Verification items for the finished model (mm, model axes). Give positions to 0.01 mm unless a question says otherwise; leave off trailing zeros. Loops run counter-clockwise (first coordinate to the right, second up) from the corner with the lowest first, then second, coordinate; pieces in that order, holes last. Notation, with made-up numbers: (63.5, -13.5) - (115.5, -13.5) arc R8 cw to (115.5, -0.5) - close; hole circle Ø10 at (46, 59). An arc over 180 degrees is marked (long way). One line per question, with ' | ' between items. Start each with the question number.
1. Section check B-B, the plane x = -57.15. Enter the section's corners in (y, z).
2. Section check C-C, the plane y = 79. Enter the section's corners in (x, z).
3. Section check A-A, the plane y = 50.8. Enter the section's corners in (x, z), then the cut area to 3 significant figures.
4. Section check D-D, the plane z = 2.5. State how many separate pieces and enclosed holes the cut face has, then the cut area to 3 significant figures.
5. Depth check by flat-ended pin: pin 1 Ø1.5 at (x, y) = (-89.5, 11.5) entering from -Z. Enter the tip coordinate at first touch or a pass-through.
6. Thickness scan on line 1 along Y through (x, z) = (-7.5, 5); line 2 along Y through (x, z) = (-57.15, 4); line 3 along Y through (x, z) = (-13.5, 1.25). Record the ranges inside material, lowest first. Write a range as from..to.
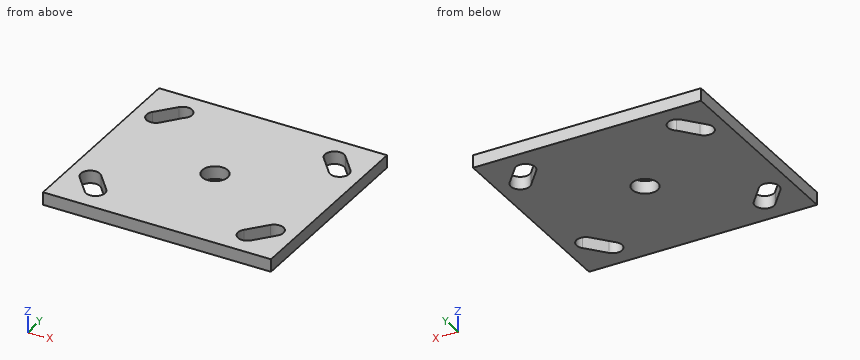
Autodesk Inventor part; units mm, degrees
ref_plane "YZ Plane" through (0, 0, 0) normal (1, 0, 0) x (0, 1, 0)
ref_plane "XZ Plane" through (0, 0, 0) normal (0, 1, 0) x (-1, 0, 0)
ref_plane "XY Plane" through (0, 0, 0) normal (0, 0, 1) x (1, 0, 0)
sketch "Sketch1" plane through (0, 0, 0) normal (0, 0, 1) x (1, 0, 0)
  line L0 (0, 0) -> (-114.3, 0)
  line L1 (-114.3, 0) -> (-114.3, 101.6)
  line L2 (-114.3, 101.6) -> (0, 101.6)
  line L3 (0, 101.6) -> (0, 0)
  line L4 (0, 50.8) -> (0, 12.7)
  line L5 (0, 50.8) -> (0, 88.9)
  line L6 (-114.3, 50.8) -> (-114.3, 88.9)
  line L7 (-114.3, 50.8) -> (-114.3, 12.7)
  arc A0 (-92.4707, 85.033) -> (-98.8773, 91.9861) centre (-95.2491, 88.9011) ccw
  arc A1 (-15.4219, 91.9851) -> (-22.6777, 85.8144) centre (-19.05, 88.9) ccw
  arc A2 (-98.8781, 9.6149) -> (-91.6219, 15.7851) centre (-95.25, 12.7) ccw
  arc A3 (-22.6781, 15.7851) -> (-15.4219, 9.6149) centre (-19.05, 12.7) ccw
  line L8 (-57.15, 0) -> (-103.1875, 0)
  line L9 (-57.15, 0) -> (-11.1125, 0)
  line L10 (-57.15, 101.6) -> (-103.1875, 101.6)
  line L11 (-57.15, 101.6) -> (-11.1125, 101.6)
  arc A4 (-99.5594, 25.1196) -> (-106.8156, 18.9494) centre (-103.1875, 22.0345) ccw
  arc A5 (-7.4844, 18.9494) -> (-14.7406, 25.1196) centre (-11.1125, 22.0345) ccw
  arc A6 (-106.8154, 82.6503) -> (-99.5202, 76.5264) centre (-103.1872, 79.5653) ccw
  arc A7 (-14.7386, 76.4804) -> (-7.4832, 82.6517) centre (-11.1109, 79.5661) ccw
  line L12 (-90.9324, 86.8892) -> (-99.5202, 76.5264)
  line L13 (-106.8154, 82.6503) -> (-98.8773, 91.9861)
  line L14 (-15.4227, 91.9861) -> (-7.4832, 82.6517)
  line L15 (-14.7386, 76.4804) -> (-22.6777, 85.8144)
  line L16 (-14.7406, 25.1196) -> (-22.6781, 15.7851)
  line L17 (-15.4219, 9.6149) -> (-7.4844, 18.9494)
  line L18 (-99.5594, 25.1196) -> (-91.6219, 15.7851)
  line L19 (-106.8156, 18.9494) -> (-98.8781, 9.6149)
  dimension "d0" = 114.3
  dimension "d1" = 101.6
  dimension "d8" = 9.525
  dimension "d9" = 9.525
  dimension "d10" = 9.525
  dimension "d11" = 46.0375
  dimension "d14" = 46.0375
  dimension "d16" = 9.525
  dimension "d20" = 9.525
  dimension "d22" = 9.525
extrude "Extrusion1" add sketch "Sketch1" along normal blind 6.35
sketch "Sketch2" plane through (0, 0, 0) normal (0, 0, -1) x (-1, 0, 0)
  line L0 (0, 101.6) -> (114.3, 101.6)
  line L1 (0, 101.6) -> (57.15, 101.6)
  line L2 (57.15, 101.6) -> (57.15, 50.8)
  circle A0 centre (57.15, 50.8) radius 6.35
  dimension "d25" = 12.7
extrude "Extrusion2" cut sketch "Sketch2" against normal blind 6.35
properties part number "wheel mount plate"
Results list:
1) outline: (0, 0) - (44.45, 0) - (44.45, 6.35) - (0, 6.35) - close; (57.15, 0) - (101.6, 0) - (101.6, 6.35) - (57.15, 6.35) - close
2) outline: (-114.3, 0) - (-107.92, 0) - (-107.92, 6.35) - (-114.3, 6.35) - close; (-97.47, 0) - (-16.88, 0) - (-16.88, 6.35) - (-97.47, 6.35) - close; (-6.38, 0) - (0, 0) - (0, 6.35) - (-6.38, 6.35) - close
3) outline: (-114.3, 0) - (-63.5, 0) - (-63.5, 6.35) - (-114.3, 6.35) - close; (-50.8, 0) - (0, 0) - (0, 6.35) - (-50.8, 6.35) - close | area: 645 mm²
4) separate pieces: 1 | enclosed holes: 5 | area: 10,700 mm²
5) pin 1: z = 0
6) line 1: 0..18.93, 25.14..76.46, 82.67..101.6 | line 2: 0..44.45, 57.15..101.6 | line 3: 0..11.88, 26.16..75.45, 89.73..101.6
